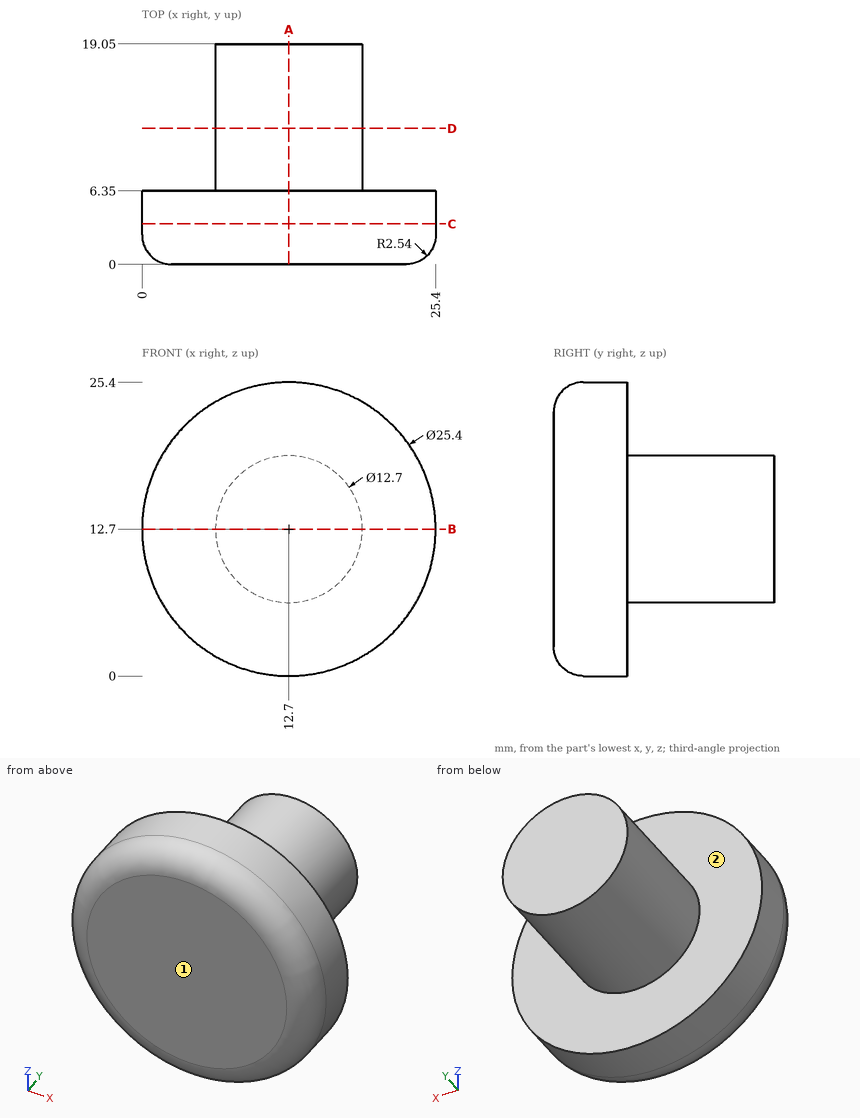
Input: dimensioned drawing with shaded views. Units: mm. Origin: part minimum x, y, z. A direction names the side the tool comes from. Coordinates: 2 decimals unless noted, no trailing zeros. Loops run counter-clockwise (first coordinate to the right, second up) from the corner with the lowest first, then second, coordinate; pieces in that order, holes last. Notation, with made-up numbers: (-23.75, 8.25) -> (30.25, 8.25) arc R31 ccw to (30.25, 36.25) -> close; hole circle Ø9 at (-8.75, 38.5). An arc over 180 degrees is marked (long way). One line per item, written item: value. Start each with the question number.
Q1. Section query C-C, the plane y = 3.5. Return the cut outline in (x, z), and give its area (3 significant figures).
Q2. Section query A-A, the plane x = 12.7. Return the cut outline in (y, z), and give its area (3 significant figures).
Q3. Section query D-D, the plane y = 11.75. Return the cut outline in (x, z).
Q4. Contact query for flat-ended pins moving along their axis: P1, Ø2, axis at y = 10, z = 7.5, coming from the +X side; P2, Ø1.5, axis at y = 12, z = 17, coming from the +X side (3 decimals); P3, Ø1, axis at x = 4.5, z = 21, coming from the -Y side. Output: stop coordinate, or through.
Q5. Line query: line 1 along Y through (x, z) = (8.25, 6); line 2 along Z through (x, y) = (12.75, 18.25); line 3 along X through (y, z) = (6.25, 22). Output: solid intervals per line, ascending.
Q6. Section query B-B, the plane z = 12.7. Return the cut outline in (x, y).
Q7. Set-up query: the marked faces 1 and 2. Return all of +Z, -Z, +X, -X, +Y, -Y with unobstructed straight access to the full face (end or side cutting, diameter ignored); none if empty.
Results:
1. outline: circle Ø25.4 at (12.7, 12.7)
1. area: 507 mm^2
2. outline: (0, 2.54) arc R2.54 ccw to (2.54, 0) -> (6.35, 0) -> (6.35, 6.35) -> (19.05, 6.35) -> (19.05, 19.05) -> (6.35, 19.05) -> (6.35, 25.4) -> (2.54, 25.4) arc R2.54 ccw to (0, 22.86) -> close
2. area: 320 mm^2
3. outline: circle Ø12.7 at (12.7, 12.7)
4. P1: x = 17.46
4. P2: x = 17.965
4. P3: y = 0.21
5. line 1: 0 to 6.35
5. line 2: 6.35 to 19.05
5. line 3: 4.05 to 21.35
6. outline: (0, 2.54) arc R2.54 ccw to (2.54, 0) -> (22.86, 0) arc R2.54 ccw to (25.4, 2.54) -> (25.4, 6.35) -> (19.05, 6.35) -> (19.05, 19.05) -> (6.35, 19.05) -> (6.35, 6.35) -> (0, 6.35) -> close
7. face 1: +Z, -Z, +X, -X, -Y
7. face 2: +Y
